from build123d import *

# Parameters (mm, degrees)
BOSS_EXTRUDE1_DEPTH = 3
SKETCH1_4_R         = 1.5
BOSS_EXTRUDE3_DEPTH = 2
SKETCH2_OUTSIDE_W   = 100.51
SKETCH2_OUTSIDE_H   = 98.431
CUT_EXTRUDE2_DEPTH  = 10


with BuildPart() as part:
    # Sketch1 → Boss-Extrude1 (new body)
    with BuildSketch(Plane(origin=(0, 0, 0), x_dir=(1, 0, 0), z_dir=(0, 1, 0))):
        with BuildLine():
            Line((-12.480384609, 34.660769231), (12.480384609, 34.660769231))
            ThreePointArc((12.480384609, 34.660769231), (0, -36.839230769), (-12.480384609, 34.660769231))
        make_face()
        with BuildLine():
            ThreePointArc((-12.5, 32.691742077), (0, -35), (12.5, 32.691742077))
            Line((12.5, 32.691742077), (-12.5, 32.691742077))
        make_face(mode=Mode.SUBTRACT)
    extrude(amount=BOSS_EXTRUDE1_DEPTH)

    # Sketch1<4> → Boss-Extrude3 (add)
    with BuildSketch(Plane(origin=(0, 0, 0), x_dir=(1, 0, 0), z_dir=(0, 1, 0))):
        with BuildLine():
            Line((12.480384609, 36.42101042), (-12.480384609, 36.42101042))
            ThreePointArc((-12.480384609, 36.42101042), (0, -38.5), (12.480384609, 36.42101042))
        make_face()
        with Locations(Location((0, 30.5, 0), (0, 0, 270))):
            Circle(SKETCH1_4_R, mode=Mode.SUBTRACT)
        with Locations(Location((4.771251184, 30.124494388, 0), (0, 0, 270))):
            Circle(SKETCH1_4_R, mode=Mode.SUBTRACT)
        with Locations(Location((9.425018328, 29.007223747, 0), (0, 0, 270))):
            Circle(SKETCH1_4_R, mode=Mode.SUBTRACT)
        with Locations(Location((13.846710242, 27.175698988, 0), (0, 0, 270))):
            Circle(SKETCH1_4_R, mode=Mode.SUBTRACT)
        with Locations(Location((17.927450195, 24.675018328, 0), (0, 0, 270))):
            Circle(SKETCH1_4_R, mode=Mode.SUBTRACT)
        with Locations(Location((21.566756826, 21.566756826, 0), (0, 0, 270))):
            Circle(SKETCH1_4_R, mode=Mode.SUBTRACT)
        with Locations(Location((24.675018328, 17.927450195, 0), (0, 0, 270))):
            Circle(SKETCH1_4_R, mode=Mode.SUBTRACT)
        with Locations(Location((27.175698988, 13.846710242, 0), (0, 0, 270))):
            Circle(SKETCH1_4_R, mode=Mode.SUBTRACT)
        with Locations(Location((29.007223747, 9.425018328, 0), (0, 0, 270))):
            Circle(SKETCH1_4_R, mode=Mode.SUBTRACT)
        with Locations(Location((30.124494388, 4.771251184, 0), (0, 0, 270))):
            Circle(SKETCH1_4_R, mode=Mode.SUBTRACT)
        with Locations(Location((30.5, 0, 0), (0, 0, 270))):
            Circle(SKETCH1_4_R, mode=Mode.SUBTRACT)
        with Locations(Location((30.124494388, -4.771251184, 0), (0, 0, 270))):
            Circle(SKETCH1_4_R, mode=Mode.SUBTRACT)
        with Locations(Location((29.007223747, -9.425018328, 0), (0, 0, 270))):
            Circle(SKETCH1_4_R, mode=Mode.SUBTRACT)
        with Locations(Location((27.175698988, -13.846710242, 0), (0, 0, 270))):
            Circle(SKETCH1_4_R, mode=Mode.SUBTRACT)
        with Locations(Location((24.675018328, -17.927450195, 0), (0, 0, 270))):
            Circle(SKETCH1_4_R, mode=Mode.SUBTRACT)
        with Locations(Location((21.566756826, -21.566756826, 0), (0, 0, 270))):
            Circle(SKETCH1_4_R, mode=Mode.SUBTRACT)
        with Locations(Location((17.927450195, -24.675018328, 0), (0, 0, 270))):
            Circle(SKETCH1_4_R, mode=Mode.SUBTRACT)
        with Locations(Location((13.846710242, -27.175698988, 0), (0, 0, 270))):
            Circle(SKETCH1_4_R, mode=Mode.SUBTRACT)
        with Locations(Location((9.425018328, -29.007223747, 0), (0, 0, 270))):
            Circle(SKETCH1_4_R, mode=Mode.SUBTRACT)
        with Locations(Location((4.771251184, -30.124494388, 0), (0, 0, 270))):
            Circle(SKETCH1_4_R, mode=Mode.SUBTRACT)
        with Locations(Location((0, -30.5, 0), (0, 0, 270))):
            Circle(SKETCH1_4_R, mode=Mode.SUBTRACT)
        with Locations(Location((-4.771251184, -30.124494388, 0), (0, 0, 270))):
            Circle(SKETCH1_4_R, mode=Mode.SUBTRACT)
        with Locations(Location((-9.425018328, -29.007223747, 0), (0, 0, 270))):
            Circle(SKETCH1_4_R, mode=Mode.SUBTRACT)
        with Locations(Location((-13.846710242, -27.175698988, 0), (0, 0, 270))):
            Circle(SKETCH1_4_R, mode=Mode.SUBTRACT)
        with Locations(Location((-17.927450195, -24.675018328, 0), (0, 0, 270))):
            Circle(SKETCH1_4_R, mode=Mode.SUBTRACT)
        with Locations(Location((-21.566756826, -21.566756826, 0), (0, 0, 270))):
            Circle(SKETCH1_4_R, mode=Mode.SUBTRACT)
        with Locations(Location((-24.675018328, -17.927450195, 0), (0, 0, 270))):
            Circle(SKETCH1_4_R, mode=Mode.SUBTRACT)
        with Locations(Location((-27.175698988, -13.846710242, 0), (0, 0, 270))):
            Circle(SKETCH1_4_R, mode=Mode.SUBTRACT)
        with Locations(Location((-29.007223747, -9.425018328, 0), (0, 0, 270))):
            Circle(SKETCH1_4_R, mode=Mode.SUBTRACT)
        with Locations(Location((-30.124494388, -4.771251184, 0), (0, 0, 270))):
            Circle(SKETCH1_4_R, mode=Mode.SUBTRACT)
        with Locations(Location((-30.5, 0, 0), (0, 0, 270))):
            Circle(SKETCH1_4_R, mode=Mode.SUBTRACT)
        with Locations(Location((-30.124494388, 4.771251184, 0), (0, 0, 270))):
            Circle(SKETCH1_4_R, mode=Mode.SUBTRACT)
        with Locations(Location((-29.007223747, 9.425018328, 0), (0, 0, 270))):
            Circle(SKETCH1_4_R, mode=Mode.SUBTRACT)
        with Locations(Location((-27.175698988, 13.846710242, 0), (0, 0, 270))):
            Circle(SKETCH1_4_R, mode=Mode.SUBTRACT)
        with Locations(Location((-24.675018328, 17.927450195, 0), (0, 0, 270))):
            Circle(SKETCH1_4_R, mode=Mode.SUBTRACT)
        with Locations(Location((-21.566756826, 21.566756826, 0), (0, 0, 270))):
            Circle(SKETCH1_4_R, mode=Mode.SUBTRACT)
        with Locations(Location((-17.927450195, 24.675018328, 0), (0, 0, 270))):
            Circle(SKETCH1_4_R, mode=Mode.SUBTRACT)
        with Locations(Location((-13.846710242, 27.175698988, 0), (0, 0, 270))):
            Circle(SKETCH1_4_R, mode=Mode.SUBTRACT)
        with Locations(Location((-9.425018328, 29.007223747, 0), (0, 0, 270))):
            Circle(SKETCH1_4_R, mode=Mode.SUBTRACT)
        with Locations(Location((-4.771251184, 30.124494388, 0), (0, 0, 270))):
            Circle(SKETCH1_4_R, mode=Mode.SUBTRACT)
        with Locations(Location((0, 25, 0), (0, 0, 270))):
            Circle(SKETCH1_4_R, mode=Mode.SUBTRACT)
        with Locations(Location((4.87725805, 24.51963201, 0), (0, 0, 270))):
            Circle(SKETCH1_4_R, mode=Mode.SUBTRACT)
        with Locations(Location((9.567085809, 23.096988313, 0), (0, 0, 270))):
            Circle(SKETCH1_4_R, mode=Mode.SUBTRACT)
        with Locations(Location((13.889255825, 20.786740308, 0), (0, 0, 270))):
            Circle(SKETCH1_4_R, mode=Mode.SUBTRACT)
        with Locations(Location((17.67766953, 17.67766953, 0), (0, 0, 270))):
            Circle(SKETCH1_4_R, mode=Mode.SUBTRACT)
        with Locations(Location((20.786740308, 13.889255825, 0), (0, 0, 270))):
            Circle(SKETCH1_4_R, mode=Mode.SUBTRACT)
        with Locations(Location((23.096988313, 9.567085809, 0), (0, 0, 270))):
            Circle(SKETCH1_4_R, mode=Mode.SUBTRACT)
        with Locations(Location((24.51963201, 4.87725805, 0), (0, 0, 270))):
            Circle(SKETCH1_4_R, mode=Mode.SUBTRACT)
        with Locations(Location((25, 0, 0), (0, 0, 270))):
            Circle(SKETCH1_4_R, mode=Mode.SUBTRACT)
        with Locations(Location((24.51963201, -4.87725805, 0), (0, 0, 270))):
            Circle(SKETCH1_4_R, mode=Mode.SUBTRACT)
        with Locations(Location((23.096988313, -9.567085809, 0), (0, 0, 270))):
            Circle(SKETCH1_4_R, mode=Mode.SUBTRACT)
        with Locations(Location((20.786740308, -13.889255825, 0), (0, 0, 270))):
            Circle(SKETCH1_4_R, mode=Mode.SUBTRACT)
        with Locations(Location((17.67766953, -17.67766953, 0), (0, 0, 270))):
            Circle(SKETCH1_4_R, mode=Mode.SUBTRACT)
        with Locations(Location((13.889255825, -20.786740308, 0), (0, 0, 270))):
            Circle(SKETCH1_4_R, mode=Mode.SUBTRACT)
        with Locations(Location((9.567085809, -23.096988313, 0), (0, 0, 270))):
            Circle(SKETCH1_4_R, mode=Mode.SUBTRACT)
        with Locations(Location((4.87725805, -24.51963201, 0), (0, 0, 270))):
            Circle(SKETCH1_4_R, mode=Mode.SUBTRACT)
        with Locations(Location((0, -25, 0), (0, 0, 270))):
            Circle(SKETCH1_4_R, mode=Mode.SUBTRACT)
        with Locations(Location((-4.87725805, -24.51963201, 0), (0, 0, 270))):
            Circle(SKETCH1_4_R, mode=Mode.SUBTRACT)
        with Locations(Location((-9.567085809, -23.096988313, 0), (0, 0, 270))):
            Circle(SKETCH1_4_R, mode=Mode.SUBTRACT)
        with Locations(Location((-13.889255825, -20.786740308, 0), (0, 0, 270))):
            Circle(SKETCH1_4_R, mode=Mode.SUBTRACT)
        with Locations(Location((-17.67766953, -17.67766953, 0), (0, 0, 270))):
            Circle(SKETCH1_4_R, mode=Mode.SUBTRACT)
        with Locations(Location((-20.786740308, -13.889255825, 0), (0, 0, 270))):
            Circle(SKETCH1_4_R, mode=Mode.SUBTRACT)
        with Locations(Location((-23.096988313, -9.567085809, 0), (0, 0, 270))):
            Circle(SKETCH1_4_R, mode=Mode.SUBTRACT)
        with Locations(Location((-24.51963201, -4.87725805, 0), (0, 0, 270))):
            Circle(SKETCH1_4_R, mode=Mode.SUBTRACT)
        with Locations(Location((-25, 0, 0), (0, 0, 270))):
            Circle(SKETCH1_4_R, mode=Mode.SUBTRACT)
        with Locations(Location((-24.51963201, 4.87725805, 0), (0, 0, 270))):
            Circle(SKETCH1_4_R, mode=Mode.SUBTRACT)
        with Locations(Location((-23.096988313, 9.567085809, 0), (0, 0, 270))):
            Circle(SKETCH1_4_R, mode=Mode.SUBTRACT)
        with Locations(Location((-20.786740308, 13.889255825, 0), (0, 0, 270))):
            Circle(SKETCH1_4_R, mode=Mode.SUBTRACT)
        with Locations(Location((-17.67766953, 17.67766953, 0), (0, 0, 270))):
            Circle(SKETCH1_4_R, mode=Mode.SUBTRACT)
        with Locations(Location((-13.889255825, 20.786740308, 0), (0, 0, 270))):
            Circle(SKETCH1_4_R, mode=Mode.SUBTRACT)
        with Locations(Location((-9.567085809, 23.096988313, 0), (0, 0, 270))):
            Circle(SKETCH1_4_R, mode=Mode.SUBTRACT)
        with Locations(Location((-4.87725805, 24.51963201, 0), (0, 0, 270))):
            Circle(SKETCH1_4_R, mode=Mode.SUBTRACT)
    extrude(amount=-BOSS_EXTRUDE3_DEPTH)

    # Sketch2 outside → Cut-Extrude2 (cut)
    with BuildSketch(Plane(origin=(0, 0, 0), x_dir=(1, 0, 0), z_dir=(0, 1, 0))):
        with Locations((0, -1.0395)):
            Rectangle(SKETCH2_OUTSIDE_W, SKETCH2_OUTSIDE_H)
        with BuildLine():
            Line((12.447023908, 36.22101042), (-12.447023908, 36.22101042))
            ThreePointArc((-12.447023908, 36.22101042), (0, -38.3), (12.447023908, 36.22101042))
        make_face(mode=Mode.SUBTRACT)
    extrude(amount=-CUT_EXTRUDE2_DEPTH, mode=Mode.SUBTRACT)


solid = part.part
Could you check a few things on this model? Use its own coordinates, in mm. Round coordinates to 2 decimals unless told otherwise and drop trailing zeros. Loops run counter-clockwise (first coordinate to the right, second up) from the corner with the lowest first, then second, coordinate; pieces in that order, holes last. Notation, with made-up numbers: (-5.5, 24.25) - (16.5, 24.25) arc R16 ccw to (16.5, 32.25) - close; hole circle Ø5 at (-1.5, 68). An arc over 180 degrees is marked (long way). Write item = value, one per line.
1) I need wall thicknesses on line 1 along X through (y, z) = (-0.8, 0); line 2 along X through (y, z) = (-0.15, -14.5); line 3 along Y through (x, z) = (-2.5, -7.5). Which ranges of each line are inside material? Lowest first, please. Write a range as from..to.
Computed:
line_1 = -38.3..-32, -29..-26.5, -23.5..23.5, 26.5..29, 32..38.3
line_2 = -35.45..-28.53, -25.83..-22.16, -19.42..19.42, 22.16..25.83, 28.53..35.45
line_3 = -2..0
2) I'm going to push flat-ended pins straight in: P1, Ø2, axis at y = 1.5, z = 29.5, coming from the -X side; P2, Ø3.5, axis at x = -9.43, z = 29.01, coming from the +Y side; P3, Ø1.5, axis at y = 1.5, z = -12, coming from the -X side. Where does each tip first touch, or does it pass through?
Computed:
P1 = -23.34
P2 = 0
P3 = -35.08
3) Imagine slicing it at B-B (x = 0). Please give me the cut outline in (y, z).
Computed:
outline = (-2, -36.22) - (0, -36.22) - (0, -34.66) - (3, -34.66) - (3, -32.69) - (0, -32.69) - (0, -32) - (-2, -32) - close; (-2, -29) - (0, -29) - (0, -26.5) - (-2, -26.5) - close; (-2, -23.5) - (0, -23.5) - (0, 23.5) - (-2, 23.5) - close; (-2, 26.5) - (0, 26.5) - (0, 29) - (-2, 29) - close; (-2, 32) - (0, 32) - (0, 35) - (3, 35) - (3, 36.84) - (0, 36.84) - (0, 38.3) - (-2, 38.3) - close
4) Imagine slicing it at C-C (y = 1.3). Please give me the cut outline in (x, z).
Computed:
outline = (-12.48, -34.66) - (12.48, -34.66) arc R36.84 ccw (long way) to start; hole (-12.5, -32.69) - (12.5, -32.69) arc R35 ccw (long way) to start
5) Imagine slicing it at A-A (z = 0). Please give me the cut outline in (x, y).
Computed:
outline = (-38.3, -2) - (-32, -2) - (-32, 0) - (-35, 0) - (-35, 3) - (-36.84, 3) - (-36.84, 0) - (-38.3, 0) - close; (-29, -2) - (-26.5, -2) - (-26.5, 0) - (-29, 0) - close; (-23.5, -2) - (23.5, -2) - (23.5, 0) - (-23.5, 0) - close; (26.5, -2) - (29, -2) - (29, 0) - (26.5, 0) - close; (32, -2) - (38.3, -2) - (38.3, 0) - (36.84, 0) - (36.84, 3) - (35, 3) - (35, 0) - (32, 0) - close
